Input: part model. Units: mm. Frame: model coordinates. Face numbers are marked on the shaded views. Round coordinates to 2 decimals unless told otherwise and drop trailing zeros. Order: outer loops, then holes, each group sorted by start corner. A loop starts at its lowest first (then second) coordinate and runs counter-clockwise, first axis right, second up. Notation, with made-up numbers: (-3, 71) -> (42, 71) arc R9 ccw to (42, 79) -> close; hole circle Ø4 at (62.25, -31). An arc over 180 degrees is marked (long way). Use a Markdown table: item, result.
from build123d import *

# Parameters (mm, degrees)
SKETCH_1_R          = 4.975
EXTRUDE_1_DEPTH     = 0.8
SKETCH_1_6_R        = 1.7
EXTRUDE_2_DEPTH     = 3.7
SKETCH_1_4_R        = 1.15
CUT_EXTRUDE_1_DEPTH = 0.5
SKETCH_1_7_R        = 1
CUT_EXTRUDE_2_DEPTH = 4.7
FILLET_1_R          = 0.2


with BuildPart() as part:
    # Sketch 1 → Extrude 1 (new body)
    with BuildSketch(Plane.XY):
        Circle(SKETCH_1_R)
    extrude(amount=EXTRUDE_1_DEPTH)

    # Sketch 1_6 → Extrude 2 (add)
    with BuildSketch(Plane.XY):
        Circle(SKETCH_1_6_R)
    extrude(amount=EXTRUDE_2_DEPTH)

    # Sketch 1_4 → Cut-Extrude 1 (cut)
    with BuildSketch(Plane.XY):
        Circle(SKETCH_1_4_R)
    extrude(amount=CUT_EXTRUDE_1_DEPTH, mode=Mode.SUBTRACT)

    # Sketch 1_7 → Cut-Extrude 2 (cut, through all)
    with BuildSketch(Plane.XY):
        with BuildLine():
            Line((-0.7, -1.549193338), (-0.7, -2.19089023))
            ThreePointArc((-0.7, -2.19089023), (0, -2.3), (0.7, -2.19089023))
            Line((0.7, -2.19089023), (0.7, -1.549193338))
            ThreePointArc((0.7, -1.549193338), (0, -1.7), (-0.7, -1.549193338))
        make_face()
        with BuildLine():
            ThreePointArc((0.7, 2.19089023), (0, 2.3), (-0.7, 2.19089023))
            Line((-0.7, 2.19089023), (-0.7, 1.549193338))
            ThreePointArc((-0.7, 1.549193338), (0, 1.7), (0.7, 1.549193338))
            Line((0.7, 1.549193338), (0.7, 2.19089023))
        make_face()
        with BuildLine():
            Line((-0.7, -1.549193338), (-0.7, -2.19089023))
            ThreePointArc((-0.7, -2.19089023), (0, -2.3), (0.7, -2.19089023))
            Line((0.7, -2.19089023), (0.7, -1.549193338))
            ThreePointArc((0.7, -1.549193338), (0, -1.7), (-0.7, -1.549193338))
        make_face()
        with BuildLine():
            ThreePointArc((0.7, 2.19089023), (0, 2.3), (-0.7, 2.19089023))
            Line((-0.7, 2.19089023), (-0.7, 1.549193338))
            ThreePointArc((-0.7, 1.549193338), (0, 1.7), (0.7, 1.549193338))
            Line((0.7, 1.549193338), (0.7, 2.19089023))
        make_face()
        Circle(SKETCH_1_7_R)
    extrude(amount=CUT_EXTRUDE_2_DEPTH, mode=Mode.SUBTRACT)

    # Fillet 1
    fillet_1_edges = [part.edges().sort_by_distance(p)[0] for p in [
        (1.428285686, 0.921954446, 3.7),
    ]]
    fillet(fillet_1_edges, radius=FILLET_1_R)


solid = part.part
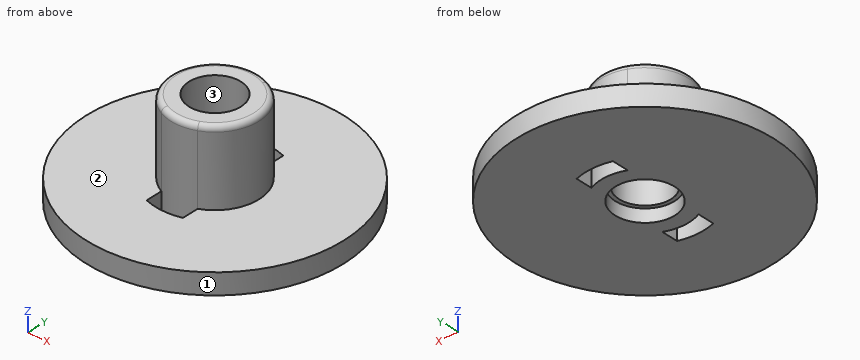
1) Line query: L1, parallel to Y at x = 0, z = 0.3 (3 decimals); L2, parallel to Y at x = 0, z = 2.65. Output: solid intervals per line, ascending. Write a range as [from, to].
Results found:
| item | result |
|---|---|
| L1 | y = [-4.975, -2.3], [-1.7, -1.15], [1.15, 1.7], [2.3, 4.975] |
| L2 | y = [-1.7, -1], [1, 1.7] |
2) Pin query (flat end, axial travel): pin 1 Ø2 at (x, y) = (-4, -3) entering from +Z; pin 2 Ø2 at (y, z) = (2.5, 3.5) entering from -X; pin 3 Ø0.7 at (y, z) = (2, 0.5) entering from -X. Return the tip coordinate at first contact, or that it passes through.
Results found:
| item | result |
|---|---|
| pin 1 | stops at z = 0.8 |
| pin 2 | stops at x = -0.8 |
| pin 3 | stops at x = -4.69 |
3) Cut plane C-C on z = 1.05. Return loops of the section in (x, y).
Results found:
| item | result |
|---|---|
| outline | circle Ø3.4 at (0, 0); hole circle Ø2 at (0, 0) |
4) Cut plane D-D on y = -2. Return loops of the section in (x, z), and give its area (3 significant figures).
Results found:
| item | result |
|---|---|
| outline | (-4.56, 0) -> (-0.7, 0) -> (-0.7, 0.8) -> (-4.56, 0.8) -> close; (0.7, 0) -> (4.56, 0) -> (4.56, 0.8) -> (0.7, 0.8) -> close |
| area | 6.17 mm² |
5) Pull-direction query (Y, two-part tool) for the marked faces 1, 2 and 3; classes: +Y half, -Y half, draft (parallel to the pull), parting line (faces both ways), or undercut.
Results found:
| item | result |
|---|---|
| face 1 | parting line |
| face 2 | draft |
| face 3 | undercut |
6) Cut plane B-B on x = 0. Return loops of the section in (y, z) (3 decimals), and give its area (3 significant figures).
Results found:
| item | result |
|---|---|
| outline | (-4.975, 0) -> (-2.3, 0) -> (-2.3, 0.8) -> (-4.975, 0.8) -> close; (-1.7, 0) -> (-1.15, 0) -> (-1.15, 0.5) -> (-1, 0.5) -> (-1, 3.7) -> (-1.5, 3.7) arc R0.2 ccw to (-1.7, 3.5) -> close; (1, 0.5) -> (1.15, 0.5) -> (1.15, 0) -> (1.7, 0) -> (1.7, 3.5) arc R0.2 ccw to (1.5, 3.7) -> (1, 3.7) -> close; (2.3, 0) -> (4.975, 0) -> (4.975, 0.8) -> (2.3, 0.8) -> close |
| area | 9.29 mm² |
7) Cut plane A-A on y = 0. Return loops of the section in (x, z) (3 decimals).
Results found:
| item | result |
|---|---|
| outline | (-4.975, 0) -> (-1.15, 0) -> (-1.15, 0.5) -> (-1, 0.5) -> (-1, 3.7) -> (-1.5, 3.7) arc R0.2 ccw to (-1.7, 3.5) -> (-1.7, 0.8) -> (-4.975, 0.8) -> close; (1, 0.5) -> (1.15, 0.5) -> (1.15, 0) -> (4.975, 0) -> (4.975, 0.8) -> (1.7, 0.8) -> (1.7, 3.5) arc R0.2 ccw to (1.5, 3.7) -> (1, 3.7) -> close |
